Can you work these out from the drawing? Everything is in mm from the part's minimum corner. A direction names the side the tool comes from. Coordinates: 2 decimals unless noted, no trailing zeros. Loops run counter-clockwise (first coordinate to the right, second up) from the corner with the lowest first, then second, coordinate; pieces in that order, holes last. Notation, with made-up numbers: (38.25, 34.25) -> (50.25, 34.25) arc R13 cw to (50.25, 42.25) -> close; hole circle Ø3 at (37, 61). An arc over 180 degrees is marked (long way). Use one line per item in the form item = value. Start each with the question number.
(1) On a 3-axis mill with a long thin cutter (end or side, diameter ignored), from which of +Z, -Z, +X, -X, +Y, -Y can I reach the whole of each face in a straight line? I mean the marked faces 4 and 5. Say none if no direction works.
(2) I'm going to push flat-ended pins straight in: pin 1 (10 mm diameter, centred on y = 7.5, z = 11, fed in from +X); pin 2 (4 mm diameter, centred on x = 20.04, z = 5, fed in from -Y). Where does each tip first touch, or does it pass through?
(3) I need wall thicknesses on line 1 (Y direction, x = 26.5, z = 8.25); line 2 (Z direction, x = 18, y = 5.5); line 3 (Z direction, x = 10, y = 0.35). Which ranges of each line are inside material? Lowest first, please. Write a range as [from, to].
(4) Imagine slicing it at D-D (z = 9.5). List the corners of the cut face in (x, y) for me (1 decimal).
(5) Imagine slicing it at C-C (z = 5). List the corners of the cut face in (x, y) for me.
(6) Imagine slicing it at A-A (x = 10). List the corners of the cut face in (y, z) for me.
(7) Imagine slicing it at B-B (z = 16.25). List the corners of the cut face in (x, y) for me (1 decimal).
(8) Thinking about a two-plate mould opening in Y: for the marked faces 1, 2 and 3, which applies, released by +Y, released by -Y, zero draft, split by the parting line, or undercut?
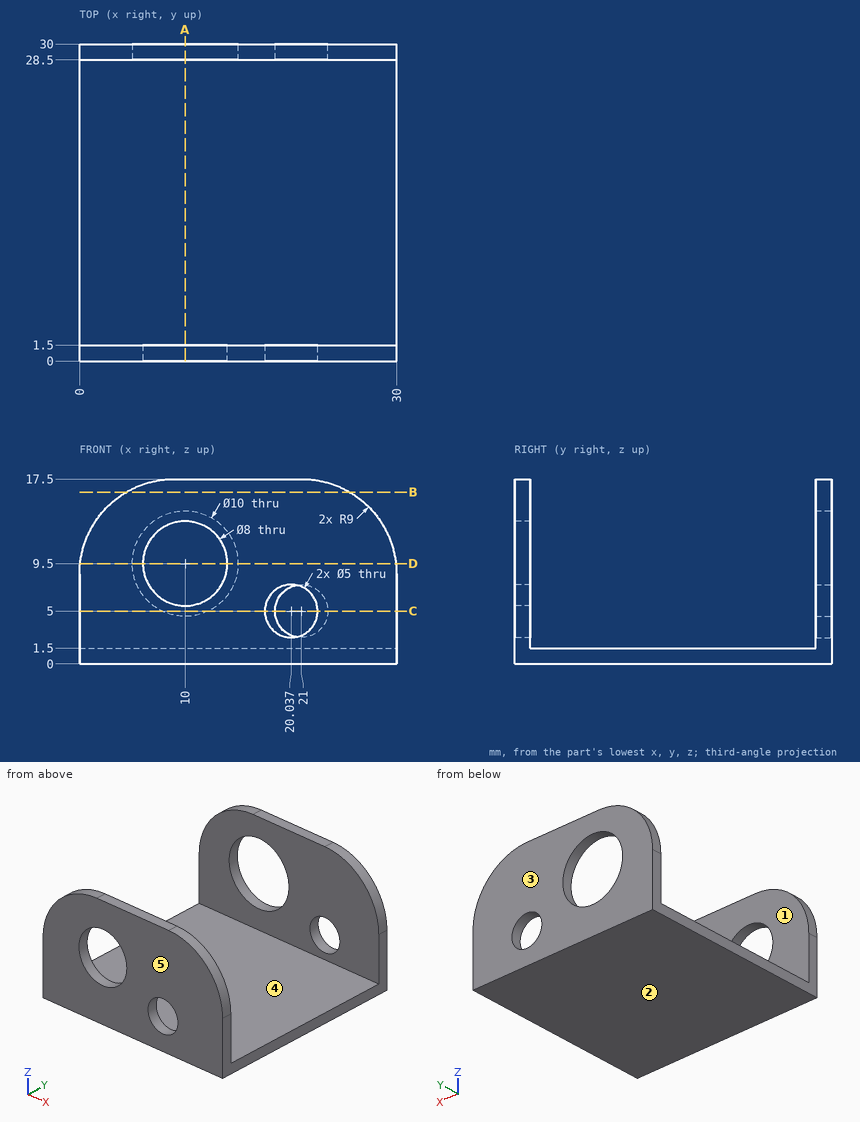
Worked out:
q1.face_4 = +Z, +X, -X
q1.face_5 = +Z, -Z, +X, -X, -Y
q2.pin_1 = through
q2.pin_2 = 28.5
q3.line_1 = [0, 1.5], [28.5, 30]
q3.line_2 = [0, 1.5]
q3.line_3 = [0, 5.5], [13.5, 17.5]
q4.outline = (0.1, 0) -> (6, 0) -> (6, 1.5) -> (0.1, 1.5) -> close; (0.1, 28.5) -> (5, 28.5) -> (5, 30) -> (0.1, 30) -> close; (14, 0) -> (29.9, 0) -> (29.9, 1.5) -> (14, 1.5) -> close; (15, 28.5) -> (29.9, 28.5) -> (29.9, 30) -> (15, 30) -> close
q5.outline = (0, 0) -> (17.54, 0) -> (17.54, 1.5) -> (0, 1.5) -> close; (0, 28.5) -> (7.82, 28.5) -> (7.82, 30) -> (0, 30) -> close; (12.18, 28.5) -> (18.5, 28.5) -> (18.5, 30) -> (12.18, 30) -> close; (22.54, 0) -> (30, 0) -> (30, 1.5) -> (22.54, 1.5) -> close; (23.5, 28.5) -> (30, 28.5) -> (30, 30) -> (23.5, 30) -> close
q6.outline = (0, 0) -> (30, 0) -> (30, 4.5) -> (28.5, 4.5) -> (28.5, 1.5) -> (1.5, 1.5) -> (1.5, 5.5) -> (0, 5.5) -> close; (0, 13.5) -> (1.5, 13.5) -> (1.5, 17.5) -> (0, 17.5) -> close; (28.5, 14.5) -> (30, 14.5) -> (30, 17.5) -> (28.5, 17.5) -> close
q7.outline = (4.4, 0) -> (25.6, 0) -> (25.6, 1.5) -> (4.4, 1.5) -> close; (4.4, 28.5) -> (25.6, 28.5) -> (25.6, 30) -> (4.4, 30) -> close
q8.face_1 = undercut
q8.face_2 = zero draft
q8.face_3 = released by +Y
